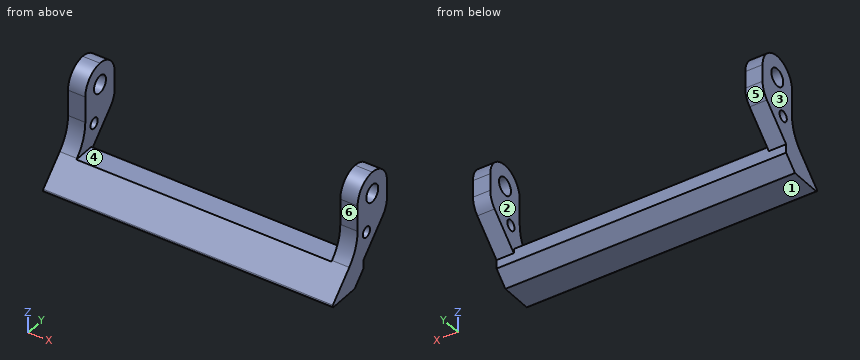
Autodesk Inventor part; units mm, degrees
ref_plane "YZ Plane" through (0, 0, 0) normal (1, 0, 0) x (0, 1, 0)
ref_plane "XZ Plane" through (0, 0, 0) normal (0, 1, 0) x (-1, 0, 0)
ref_plane "XY Plane" through (0, 0, 0) normal (0, 0, 1) x (1, 0, 0)
sketch "Skizze1" plane through (0, 0, 0) normal (1, 0, 0) x (0, 1, 0)
  line L0 (-4.8284, 6.1716) -> (-10.5, 0.5)
  line L1 (-10.5, 0) -> (-3, 0)
  line L2 (-10.5, 0.5) -> (-10.5, 0)
  line L3 (0, 5) -> (8, 13)
  circle A0 centre (3, 19) radius 0.5
  line L4 (-2, 13) -> (-2, 24)
  line L5 (-2, 24) -> (8, 24)
  line L6 (8, 24) -> (8, 13)
  line L7 (0, 3) -> (-3, 0)
  line L8 (8, 13) -> (-2, 13) construction
  arc A1 (-4.8284, 6.1716) -> (-2, 13) centre (-11.6569, 13) ccw
  line L9 (0, 5) -> (0, 3)
  line L10 (3, 19) -> (3, 0) construction
  point P0 (0, 0)
  dimension "d40" = 0.5
  dimension "d44" = 1
  dimension "d59" = 10
  dimension "d60" = 45
  dimension "d61" = 5
  dimension "d63" = 45
  dimension "d78" = 3
  dimension "d79" = 10.5
  dimension "d80" = 0
  dimension "d81" = 19
  dimension "d82" = 5
  dimension "d83" = 3
extrude "Extrusion1" add sketch "Skizze1" along normal mid plane 67
sketch "Skizze6" plane through (0, 0, 0) normal (0, 1, 0) x (-1, 0, 0)
  line L0 (33.5, 0.5) -> (-33.5, 0.5)
  line L1 (-33.5, 6.1716) -> (-33.5, 0.5)
  line L2 (33.5, 0.5) -> (33.5, 6.1716)
  line L3 (-29.5, 6) -> (29.5, 6)
  line L4 (29.5, 6) -> (29.5, 36)
  line L5 (29.5, 36) -> (-29.5, 36)
  line L6 (-29.5, 36) -> (-29.5, 6)
  line L7 (0, -7.2) -> (0, 43.2)
  line L8 (33.5, 0) -> (-33.5, 0)
  line L9 (-33.5, 0) -> (33.5, 0)
  point P0 (0, 0)
  point P1 (-33, 10)
  point P2 (33, 10)
  dimension "d45" = 4
  dimension "d46" = 30
  dimension "d50" = 6
extrude "Extrusion4" cut sketch "Skizze6" along normal through all both and the other way through all
sketch "Skizze3" plane through (-33.5, 0, 0) normal (-1, 0, 0) x (0, 0, 1)
  line L0 (0, -3) -> (0, -10.5)
  line L1 (0.5, -10.5) -> (6.1716, -4.8284)
  line L2 (0, -10.5) -> (0, 0) construction
  line L3 (0, 11.9314) -> (0, -15.5882)
  line L4 (0, -10.5) -> (0.5, -10.5)
  line L5 (13, 8) -> (5, 0)
  line L6 (13, -2) -> (24, -2)
  line L7 (24, -2) -> (24, 8)
  line L8 (24, 8) -> (13, 8)
  circle A0 centre (19, 3) radius 0.5
  line L9 (3, 0) -> (0, -3)
  arc A1 (13, -2) -> (6.1716, -4.8284) centre (13, -11.6569) ccw
  line L10 (5, 0) -> (3, 0)
hole "Bohrung1" at (-33.5, 3, 19) direction (1, 0, 0) diameter 4.05 end through all
sketch "Skizze4" plane through (-33.5, 0, 0) normal (-1, 0, 0) x (0, 0, 1)
  line L0 (0, 11.7) -> (0, -14.2)
  line L1 (-5.8, 0) -> (34.8, 0)
  point P0 (29, 0)
  point P1 (11, 1)
  dimension "d38" = 11
  dimension "d84" = 1
hole "Bohrung2" at (-33.5, 1, 11) direction (1, 0, 0) diameter 2.459 end through all
fillet "Rundung2" radius 5 6 edges at (31.5, -2, 24) (31.5, 8, 24) (-31.5, 8, 24) (-31.5, -2, 24) (31.5, 8, 13) (-31.5, 8, 13)
fillet "Rundung7" [suppressed]
fillet "Rundung8" radius 0.36 2 edges at (0, -10.5, 0.5) (0, -10.5, 0)
sketch "Skizze7" plane through (-29.5, 1, 6) normal (0, 0, 1) x (1, 0, 0)
  line L0 (0, 0) -> (59, 0)
  line L1 (0, 0) -> (0, -6)
  line L2 (59, -6) -> (0, -6)
  line L3 (59, -6) -> (59, 0)
  line L4 (-17.4, -1) -> (76.4, -1)
  point P0 (29.5, -1)
  point P1 (0, -1)
  point P2 (59, -1)
extrude "Extrusion5" cut sketch "Skizze7" against normal through all contours L0 L3 L4 L1
properties part number "Chip Schaufel v2" material "Aluminium 6061"
The listing builds one solid part. Answer for the finished solid, in the listing's coordinates (mm). Face numbers are marked on the shaded views. A direction names the side the tool comes from. Coordinates: 2 decimals unless noted, no trailing zeros. Write each loop counter-clockwise with the first axis right and the second up, starting at its lowest first coordinate (ties: lowest second). Pieces come first, ordered by that corner, then holes. Notation, with made-up numbers: (66.5, -35.75) - (87.5, -35.75) arc R25 cw to (87.5, 0.25) - close; hole circle Ø5 at (68.5, 89.25). An arc over 180 degrees is marked (long way). Return JSON: item names as keys, results as strings.
1. Each of these flat-tipped pins is pushed along its axis until it touches: pin 1 Ø2 at (x, y) = (-9.5, 2.5) entering from -Z; pin 2 Ø10 at (x, y) = (12, -2) entering from +Z; pin 3 Ø2.5 at (x, z) = (-11, 4.5) entering from +Y; pin 4 Ø4.5 at (x, z) = (30.5, 15) entering from -Y. Where does it stop, or does it pass through?
Final values:
{"pin 1": "through", "pin 2": "z = 6", "pin 3": "y = 0", "pin 4": "y = -2"}
2. The part is cut by section A-A on z = 7. Determine the outline of the cut face in (x, y).
Final values:
{"outline": "(-33.5, -4.09) - (-29.5, -4.09) - (-29.5, 2) - (-33.5, 2) - close; (29.5, -4.09) - (33.5, -4.09) - (33.5, 2) - (29.5, 2) - close"}
3. The part is cut by section B-B on x = 2.5. Determine the outline of the cut face in (y, z).
Final values:
{"outline": "(-10.5, 0.36) arc R0.36 ccw to (-10.14, 0) - (-3, 0) - (0, 3) - (0, 6) - (-5, 6) - (-10.39, 0.61) arc R0.36 ccw to start"}
4. Which of the six approach directions +Z, -Z, +X, -X, +Y, -Y give full straight-line access (tool end or side, diameter ignored) to the marked faces 4, 5 and 6?
Final values:
{"face 4": "+Z, +Y, -Y", "face 5": "-Z, +X, -X, +Y", "face 6": "+Z, +X, -X, -Y"}
5. Consider line 1 along X through (y, z) = (2.25, 23); line 2 along Z through (x, y) = (32.6, 3) (3 decimals); line 3 along Y through (x, z) = (-30.7, 19) (3 decimals). Determine where each line is inside the solid, lowest interval first.
Final values:
{"line 1": "-33.5 to -29.5, 29.5 to 33.5", "line 2": "8 to 16.975, 21.025 to 24", "line 3": "-2 to 0.975, 5.025 to 8"}
6. The part is cut by section C-C on y = 7.25. Determine the outline of the cut face in (x, z), then the cut area to 3 significant figures.
Final values:
{"outline": "(-33.5, 12.44) - (-29.5, 12.44) - (-29.5, 21.63) - (-33.5, 21.63) - close; (29.5, 12.44) - (33.5, 12.44) - (33.5, 21.63) - (29.5, 21.63) - close", "area": "73.6 mm^2"}
7. For a pull along X with two mould halves and no side action, classify the marked faces 1, 2 and 3 as +X half, -X half, draft (parallel to the pull), parting line (faces both ways), or undercut.
Final values:
{"face 1": "draft", "face 2": "undercut", "face 3": "-X half"}
